from build123d import *

# Parameters (mm, degrees)
BOSS_EXTRUDE1_DEPTH = 47
SKETCH2_R           = 1.5
CUT_EXTRUDE1_DEPTH  = 4
SKETCH3_R           = 8
CUT_EXTRUDE2_DEPTH  = 9.560785614


with BuildPart() as part:
    # Sketch1 → Boss-Extrude1 (new body)
    with BuildSketch(Plane(origin=(0, 0, 0), x_dir=(1, 0, 0), z_dir=(0, 1, 0))):
        with BuildLine():
            Line((-2.32059976, 10.913457617), (11.001200978, 10.913457617))
            ThreePointArc((11.001200978, 10.913457617), (14.215139026, 9.743679833), (15.925239743, 6.781698506))
            Line((15.925239743, 6.781698506), (20.843268829, -21.10983044))
            Line((20.843268829, -21.10983044), (17.88884557, -21.630774973))
            Line((17.88884557, -21.630774973), (13.407940849, 3.781698506))
            ThreePointArc((13.407940849, 3.781698506), (11.697840132, 6.743679833), (8.483902084, 7.913457617))
            Line((8.483902084, 7.913457617), (-2.32059976, 7.913457617))
            Line((-2.32059976, 7.913457617), (-2.32059976, 10.913457617))
        make_face()
    extrude(amount=BOSS_EXTRUDE1_DEPTH)

    # Sketch2 → Cut-Extrude1 (cut, through all)
    with BuildSketch(Plane.XY.offset(-7.913457617)):
        with Locations((2.67940024, 30)):
            Circle(SKETCH2_R)
        with Locations((2.67940024, 17)):
            Circle(SKETCH2_R)
    extrude(amount=-CUT_EXTRUDE1_DEPTH, mode=Mode.SUBTRACT)

    # Sketch3 → Cut-Extrude2 (cut, through all)
    with BuildSketch(Plane(origin=(13.650350495, 0, -2.406925088), x_dir=(0.173648178, 0, 0.984807753), z_dir=(-0.984807753, 0, 0.173648178))):
        with BuildLine():
            Line((24.408520331, 47), (13.408520331, 47))
            ThreePointArc((13.408520331, 47), (21.186694924, 43.778174593), (24.408520331, 36))
            Line((24.408520331, 36), (24.408520331, 47))
        make_face()
        with BuildLine():
            Line((24.408520331, 0), (24.408520331, 11))
            ThreePointArc((24.408520331, 11), (21.186694924, 3.221825407), (13.408520331, 0))
            Line((13.408520331, 0), (24.408520331, 0))
        make_face()
        with Locations((13.408520331, 11)):
            Circle(SKETCH3_R)
        with Locations((13.408520331, 36)):
            Circle(SKETCH3_R)
        with BuildLine():
            Line((24.408520331, 11), (24.408520331, 36))
            ThreePointArc((24.408520331, 36), (22.930853605, 30.493170692), (18.894853235, 26.465842918))
            ThreePointArc((18.894853235, 26.465842918), (17.17968635, 23.5), (18.894853235, 20.534157082))
            ThreePointArc((18.894853235, 20.534157082), (22.930853605, 16.506829308), (24.408520331, 11))
        make_face()
    extrude(amount=-CUT_EXTRUDE2_DEPTH, mode=Mode.SUBTRACT)


solid = part.part
Can you work these out from the model? Positions are in its coordinate system, mm. A direction names the side the tool comes from. Give positions to 0.01 mm unless a question says otherwise; leave off trailing zeros. Loops run counter-clockwise (first coordinate to the right, second up) from the corner with the lowest first, then second, coordinate; pieces in that order, holes last. Notation, with made-up numbers: (70.5, -12.75) -> (113.5, -12.75) arc R26 cw to (113.5, 21.25) -> close; hole circle Ø8 at (17.25, -32.5). An arc over 180 degrees is marked (long way). Write item = value, one per line.
1) Suppose I cut it at D-D on y = 23.5. Write out the boundary of the cut face in (x, z), then the cut area to 3 significant figures.
Check result:
outline = (-2.32, -10.91) -> (11, -10.91) arc R5 ccw to (15.93, -6.78) -> (19.59, 13.99) -> (16.63, 14.51) -> (13.41, -3.78) arc R5 cw to (8.48, -7.91) -> (-2.32, -7.91) -> close
area = 121 mm2
2) Thinking about a two-plate mould opening in Y: for faces 3 (the flat face through (13, 47, -6)), 4 (the cylindrical face through (17.254, 43.932, 9.515)), 5 (the flat face through (15.182, 23.171, 6.279)), which applies, released by +Y, released by -Y, zero draft, split by the parting line, or undercut?
Check result:
face_3 = released by +Y
face_4 = undercut
face_5 = zero draft
3) Suppose I cut it at A-A on y = 13. Write out the boundary of the cut face in (x, z).
Check result:
outline = (-2.32, -10.91) -> (11, -10.91) arc R5 ccw to (15.93, -6.78) -> (17.59, 2.65) -> (14.63, 3.17) -> (13.41, -3.78) arc R5 cw to (8.48, -7.91) -> (-2.32, -7.91) -> close; (17.32, 18.43) -> (20.28, 17.91) -> (20.81, 20.93) -> (17.86, 21.45) -> close
4) Will these pins go through, and if not, where does the flat tip stop? pin 1 (3 mm diameter, centred on y = 34, z = -7, fed in from +X); pin 2 (4 mm diameter, centred on y = 23.5, z = 13.5, fed in from +X); pin 3 (10 mm diameter, centred on y = 33.5, z = 8, fed in from -X).
Check result:
pin_1 = 16.15
pin_2 = 19.67
pin_3 = 14.6
5) I need wall thicknesses on L1, parallel to Z at x = 7, y = 16; L2, parallel to Z at x = 15.5, y = 33.5; L3, parallel to X at y = 3, z = 16. Which ranges of each line are inside material? Lowest first, please. Write a range as from..to.
Check result:
L1 = -10.91..-7.91
L2 = -8.1..3.17
L3 = 16.9..19.94
6) Suppose I cut it at B-B on y = 33. Write out the boundary of the cut face in (x, z).
Check result:
outline = (-2.32, -10.91) -> (11, -10.91) arc R5 ccw to (15.93, -6.78) -> (17.65, 2.97) -> (14.69, 3.49) -> (13.41, -3.78) arc R5 cw to (8.48, -7.91) -> (-2.32, -7.91) -> close; (17.27, 18.1) -> (20.22, 17.58) -> (20.77, 20.7) -> (17.82, 21.22) -> close
7) For faces 1 (the flat face through (3, 23, -7.913)), 2 (the cylindrical face through (1.57, 18.01, -9.39)), which set-ups out of +Z, -Z, +X, -X, +Y, -Y let a thin tool reach every point of the face, with its end or its side?
Check result:
face_1 = +Z, -X, +Y, -Y
face_2 = +Z, -Z
8) Suppose I cut it at C-C on x = 5.5. Write out the boundary of the cut face in (y, z).
Check result:
outline = (0, -10.91) -> (47, -10.91) -> (47, -7.91) -> (0, -7.91) -> close
